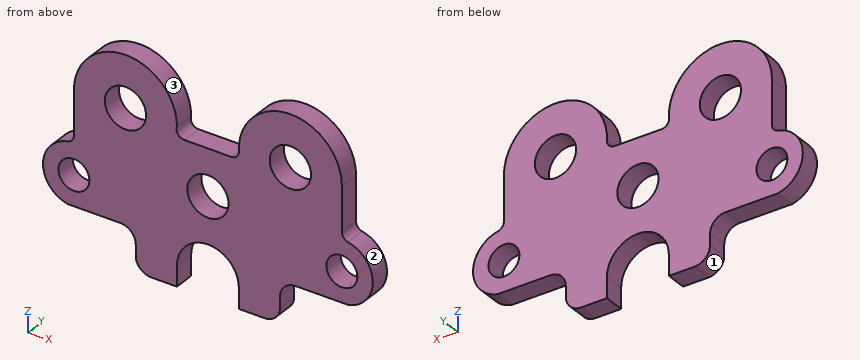
```python
from build123d import *

# Parameters (mm, degrees)
F0_R     = 9.525
F0_R_2   = 12.7
F1_DEPTH = 12.7


with BuildPart() as f1:
    # F0 (on Front) → F1 (new body)
    with BuildSketch(Plane.XZ):
        with BuildLine():
            ThreePointArc((19.080032, 33.544383), (17.7775, 30.059917), (14.366766, 28.575))
            Line((14.366766, 28.575), (-14.366766, 28.575))
            ThreePointArc((-14.366766, 28.575), (-18.355036, 30.487573), (-19.050075, 34.855771))
            ThreePointArc((-19.050075, 34.855771), (-50.765385, 66.674981), (-82.55, 34.925))
            Line((-82.55, 34.925), (-82.55, 7.45639))
            ThreePointArc((-82.55, 7.45639), (-83.623483, 4.44432), (-86.36, 2.790112))
            ThreePointArc((-86.36, 2.790112), (-101.6, -15.875), (-86.36, -34.540112))
            Line((-86.36, -34.540112), (-53.975, -34.540112))
            ThreePointArc((-53.975, -34.540112), (-47.239808, -37.32992), (-44.45, -44.065112))
            Line((-44.45, -44.065112), (-44.45, -50.8))
            ThreePointArc((-44.45, -50.8), (-41.660192, -57.535192), (-34.925, -60.325))
            Line((-34.925, -60.325), (-19.05, -60.325))
            Line((-19.05, -60.325), (-19.05, -47.625))
            ThreePointArc((-19.05, -47.625), (-13.470384, -34.154616), (0, -28.575))
            ThreePointArc((0, -28.575), (13.470384, -34.154616), (19.05, -47.625))
            Line((19.05, -47.625), (19.05, -60.325))
            Line((19.05, -60.325), (34.925, -60.325))
            ThreePointArc((34.925, -60.325), (41.660192, -57.535192), (44.45, -50.8))
            Line((44.45, -50.8), (44.45, -44.065112))
            ThreePointArc((44.45, -44.065112), (47.239808, -37.32992), (53.975, -34.540112))
            Line((53.975, -34.540112), (86.36, -34.540112))
            ThreePointArc((86.36, -34.540112), (101.6, -15.875), (86.36, 2.790112))
            ThreePointArc((86.36, 2.790112), (83.623483, 4.44432), (82.55, 7.45639))
            Line((82.55, 7.45639), (82.55, 34.925))
            ThreePointArc((82.55, 34.925), (50.109528, 66.667491), (19.080032, 33.544383))
        make_face()
        with Locations((-82.55, -15.875)):
            Circle(F0_R, mode=Mode.SUBTRACT)
        Circle(F0_R_2, mode=Mode.SUBTRACT)
        with Locations((82.55, -15.875)):
            Circle(F0_R, mode=Mode.SUBTRACT)
        with Locations((-50.8, 34.925)):
            Circle(F0_R_2, mode=Mode.SUBTRACT)
        with Locations((50.8, 34.925)):
            Circle(F0_R_2, mode=Mode.SUBTRACT)
    extrude(amount=F1_DEPTH)


solid = f1.part
```
Work out the finished part from the listing and answer in its coordinate system (mm). Face numbers are marked on the shaded views. Round coordinates to 2 decimals unless told otherwise and drop trailing zeros. Order: outer loops, then holes, each group sorted by start corner. A loop starts at its lowest first (then second) coordinate and runs counter-clockwise, first axis right, second up.
Q1. A cutting plane is placed at C-C, the plane z = -38. Determine the outline of the cut face in (x, y).
Solution:
outline: (-46.63, -12.7) - (-16.44, -12.7) - (-16.44, 0) - (-46.63, 0) - close; (16.44, -12.7) - (46.63, -12.7) - (46.63, 0) - (16.44, 0) - close
Q2. A cutting plane is placed at B-B, the plane x = 61.5. Determine the outline of the cut face in (y, z), then the cut area to 3 significant figures.
Solution:
outline: (-12.7, -34.54) - (0, -34.54) - (0, 28.08) - (-12.7, 28.08) - close; (-12.7, 41.77) - (0, 41.77) - (0, 64.82) - (-12.7, 64.82) - close
area: 1,090 mm2
Q3. A cutting plane is placed at D-D, the plane y = -6.25. Count the separate pieces of the cut face and the enclosed holes in it, then the cut area to 3 significant figures.
Solution:
separate pieces: 1
enclosed holes: 5
area: 14,700 mm2
Q4. A cutting plane is placed at A-A, the plane z = 39. Determine the outline of the cut face in (x, y).
Solution:
outline: (-82.29, -12.7) - (-62.83, -12.7) - (-62.83, 0) - (-82.29, 0) - close; (-38.77, -12.7) - (-19.31, -12.7) - (-19.31, 0) - (-38.77, 0) - close; (19.31, -12.7) - (38.77, -12.7) - (38.77, 0) - (19.31, 0) - close; (62.83, -12.7) - (82.29, -12.7) - (82.29, 0) - (62.83, 0) - close
Q5. Find the intervals of material crossed by line 1 along X through (y, z) = (-5.5, 41); line 2 along Z through (x, y) = (0, -8) (3 decimals); line 3 along X through (y, z) = (-6.25, -50.5), in increasing order.
Solution:
line 1: x = -81.96 to -61.95, -39.65 to -19.64, 19.64 to 39.65, 61.95 to 81.96
line 2: z = -28.575 to -12.7, 12.7 to 28.575
line 3: x = -44.45 to -19.05, 19.05 to 44.45
Q6. The mould has two halves that part along X. Classify the marked faces 1, 2 and 3: pulls with the +X half, pulls with the -X half, needs draft (parallel to the pull), parting line crosses it, or undercut.
Solution:
face 1: pulls with the -X half
face 2: pulls with the +X half
face 3: undercut
Q7. Given pin 1 Ø4 at (x, y) = (-70.5, -2) entering from +Z; pin 2 Ø6.5 at (x, y) = (-6.5, -9) entering from +Z (3 decimals); pin 3 Ø3.5 at (y, z) = (-3.5, -49) entering from +X; pin 4 Ø20.5 at (x, z) = (-50.8, 34.925) entering from -Y, each flat-ended and moving along its own axis, determine where each tip first touches the part or whether it passes through.
Solution:
pin 1: stops at z = 61.28
pin 2: stops at z = 28.575
pin 3: stops at x = 44.45
pin 4: passes through
